Build history of the part. All positions in model axes, mm. Face numbers are marked on the shaded views. A direction names the side the tool comes from. Round coordinates to 2 decimals unless told otherwise and drop trailing zeros. Write each loop counter-clockwise with the first axis right and the second up, starting at its lowest first coordinate (ties: lowest second). Pieces come first, ordered by that corner, then holes. Notation, with made-up numbers: (67, 31.5) -> (103, 31.5) arc R6 cw to (103, 40.5) -> close; hole circle Ø7 at (47.5, -1.5). An arc over 180 degrees is marked (long way). Answer in a Markdown table with one row per item.
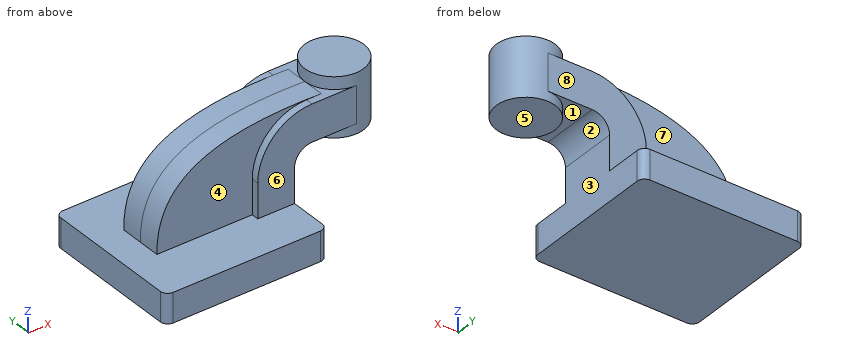
```python
from build123d import *

# Parameters (mm, degrees)
F1_DEPTH = 63.5
F0_W     = 25.4
F0_H     = 31.75
F2_DEPTH = 25.4
F3_DEPTH = 19.05
F5_R     = 6.35


with BuildPart() as f1:
    # F0 (on Front) → F1 (new body, symmetric)
    with BuildSketch(Plane.XZ):
        Polygon((-69.85, -12.7), (69.85, -12.7), (69.85, 12.7), (38.1, 12.7), (-44.13639, 12.7), (-69.85, 12.7), align=None)
    extrude(amount=F1_DEPTH, both=True)

    # F0 (on Front) → F2 (join, symmetric)
    with BuildSketch(Plane.XZ):
        with BuildLine():
            Line((38.1, 12.7), (69.85, 12.7))
            Line((69.85, 12.7), (69.85, 42.418495))
            ThreePointArc((69.85, 42.418495), (74.270896, 53.091481), (84.943882, 57.512377))
            Line((84.943882, 57.512377), (97.725361, 57.512377))
            Line((97.725361, 57.512377), (97.725361, 89.262377))
            Line((97.725361, 89.262377), (84.943882, 89.262377))
            ThreePointArc((84.943882, 89.262377), (51.820255, 75.542121), (38.1, 42.418495))
            Line((38.1, 42.418495), (38.1, 12.7))
        make_face()
        with Locations((110.425361, 73.387377)):
            Rectangle(F0_W, F0_H)
    extrude(amount=F2_DEPTH, both=True)

    # F0 (on Front) → F3 (join, symmetric)
    with BuildSketch(Plane.XZ):
        with BuildLine():
            Line((-44.13639, 12.7), (38.1, 12.7))
            Line((38.1, 12.7), (38.1, 42.418495))
            ThreePointArc((38.1, 42.418495), (51.820255, 75.542121), (84.943882, 89.262377))
            Line((84.943882, 89.262377), (97.725361, 89.262377))
            add(Edge.make_bspline(
                [(-44.13639, 12.7), (-45.473855, 76.681405), (13.374661, 92.285179), (97.725361, 89.262377)],
                knots=[0, 0, 0, 0, 161.203455, 161.203455, 161.203455, 161.203455], degree=3))
        make_face()
    extrude(amount=F3_DEPTH, both=True)

    # F0 (on Front) → F4 (revolve)
    with BuildSketch(Plane.XZ):
        Polygon((123.125361, 99.877948), (123.125361, 89.262377), (123.125361, 57.512377), (123.125361, 49.077948), (148.525361, 49.077948), (148.525361, 99.877948), align=None)
    revolve(axis=Axis((123.125361, 0, 74.477948), (0, 0, 1)))

    # F5
    f5_edges = [f1.edges().sort_by_distance(p)[0] for p in [
        (-69.85, 63.5, 0),
        (69.85, 63.5, 0),
        (-69.85, -63.5, 0),
        (69.85, -63.5, 0),
    ]]
    fillet(f5_edges, radius=F5_R)


solid = f1.part
```
Q1. Saw through at A-A on x = 107. Write the cut outline in (y, z), plus the area to 3 significant figures.
A:
| item | result |
|---|---|
| outline | (-25.4, 57.51) -> (-19.62, 57.51) -> (-19.62, 49.08) -> (19.62, 49.08) -> (19.62, 57.51) -> (25.4, 57.51) -> (25.4, 89.26) -> (19.62, 89.26) -> (19.62, 99.88) -> (-19.62, 99.88) -> (-19.62, 89.26) -> (-25.4, 89.26) -> close |
| area | 2,360 mm² |
Q2. Wall check: line 1 (Y direction, x = 107, z = 74.5); line 2 (Z direction, x = -14.5, y = 45); line 3 (Z direction, x = 127.5, y = 12.5). Give the ranges that are in metal, low to high. Write a range as [from, to].
A:
| item | result |
|---|---|
| line 1 | [-25.4, 25.4] |
| line 2 | [-12.7, 12.7] |
| line 3 | [49.08, 99.88] |
Q3. Saw through at B-B on y = -43. Write the cut outline in (x, z).
A:
| item | result |
|---|---|
| outline | (-69.85, -12.7) -> (69.85, -12.7) -> (69.85, 12.7) -> (-69.85, 12.7) -> close |
Q4. Two-plate mould, pull along X, no slides. Class the marked faces 1, 2, 3 and 4: released by +X, released by -X, zero draft, split by the parting line, or undercut.
A:
| item | result |
|---|---|
| face 1 | undercut |
| face 2 | undercut |
| face 3 | released by +X |
| face 4 | zero draft |
Q5. Which spindle directions (+Z, -Z, +X, -X, +Y, -Y) get a long thin tool onto all of the face, cutting with end or side? Do the marked faces 5, 6, 7 and 8. Say none if no direction does.
A:
| item | result |
|---|---|
| face 5 | -Z, +X, +Y, -Y |
| face 6 | +Z, +X, -X, -Y |
| face 7 | +Z, -X, +Y |
| face 8 | +Z, +X, -X, +Y |
Q6. Drop flat-ended pins along their axis: P1, Ø1.5, axis at x = 118.5, z = 80, coming from the +Y side; P2, Ø12, axis at y = 28.5, z = 54, coming from the +X side; P3, Ø12, axis at y = -37, z = 84.5, coming from the +X side; P4, Ø3, axis at y = -21.5, z = 30, coming from the -X side. Give the stop position or say it passes through.
A:
| item | result |
|---|---|
| P1 | y = 25.4 |
| P2 | x = 134.91 |
| P3 | through |
| P4 | x = 38.1 |
